Source: three-view drawing plus pictorial views. Frame: mm from the lowest corner of the part. Coordinates: 2 decimals unless noted, no trailing zeros. Write each loop counter-clockwise with the first axis right and the second up, starting at its lowest first coordinate (ties: lowest second). Pieces come first, ordered by that corner, then holes. Notation, with made-up numbers: M 20,37.25 L 75,37.25 A20 ccw 75,61.25 Z; hole C -4,-21 d6. An arc over 180 degrees is marked long. Write item = value, one per line. Start each with the question number.
Item 1: Ray query, L1, parallel to Y at x = 3, z = 192; L2, parallel to Z at x = 5.75, y = 460. Return the intervals inside material, ascending. Write a range as [from, to].
Item 2: Section A-A on y = 460. Output: boundary loops of the cut face in (x, z).
Item 3: Section B-B on z = 192. Output: boundary loops of the cut face in (x, y), plus the area to 3 significant figures.
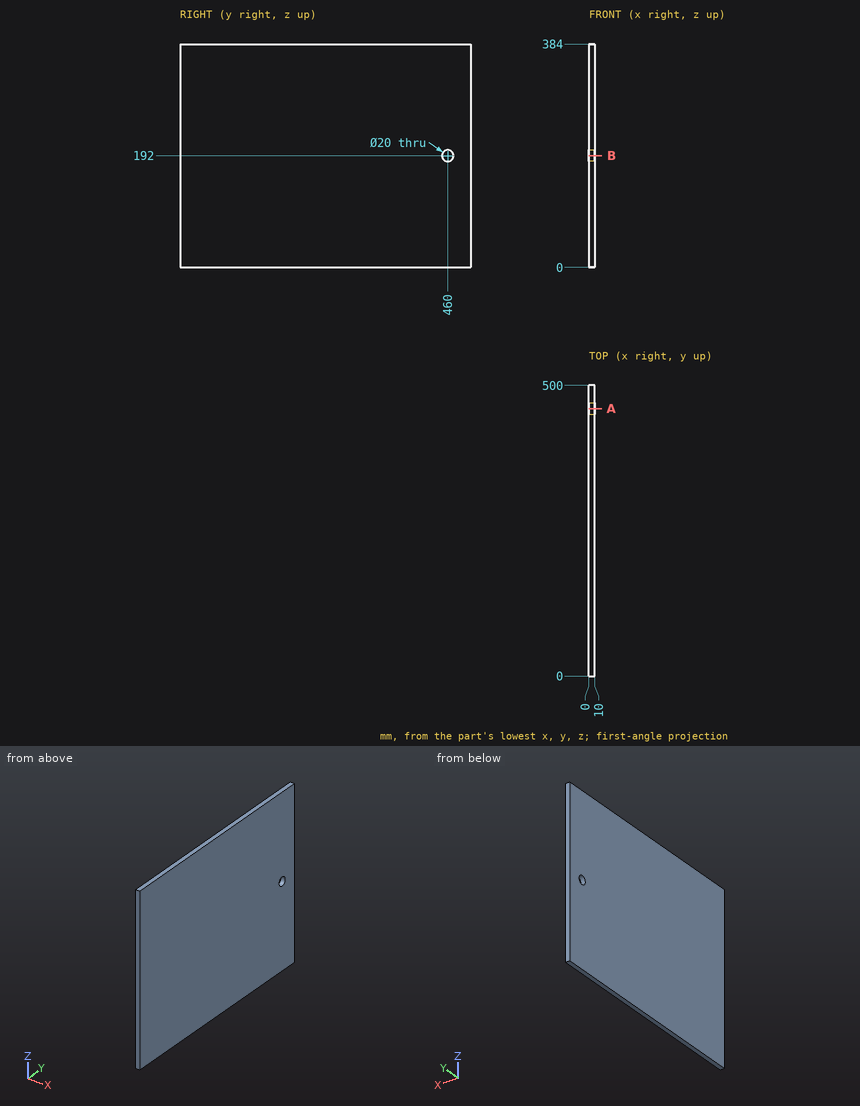
Responses:
q1.L1 = [0, 450], [470, 500]
q1.L2 = [0, 182], [202, 384]
q2.outline = M 0,0 L 10,0 L 10,182 L 0,182 Z; M 0,202 L 10,202 L 10,384 L 0,384 Z
q3.outline = M 0,0 L 10,0 L 10,450 L 0,450 Z; M 0,470 L 10,470 L 10,500 L 0,500 Z
q3.area = 4,800 mm²
